Could you check a few things on this model? Use its own coordinates, in mm. Face numbers are marked on the shaded views. A direction names the side the tool comes from. Give positions to 0.01 mm unless a question says otherwise; leave off trailing zeros. Write each loop counter-clockwise with the first axis right and the second up, starting at its lowest first coordinate (ties: lowest second). Pieces come first, ordered by that corner, then holes. Notation, with made-up numbers: M -35,-34 L -5,-34 A24 ccw -5,-3 Z; hole C 68,-23 d7. An arc over 180 degrees is marked long. Write each question's results on one line, items separated by ' | '. Start each with the question number.
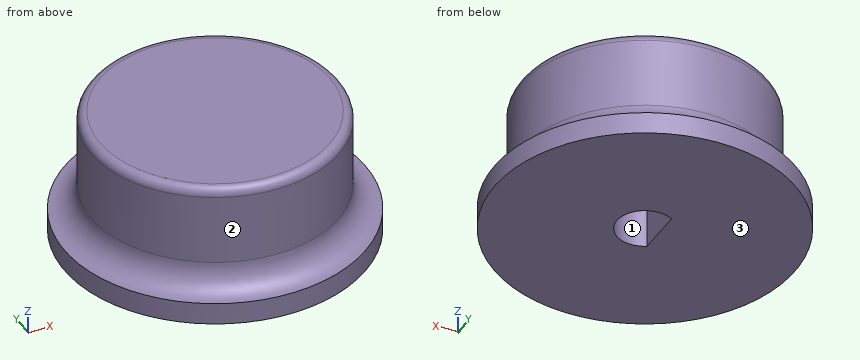
Autodesk Fusion 360 part; units mm, degrees
sketch "Sketch1" plane through (0, 0, 0) normal (0, 0, 1) x (1, 0, 0)
  line L0 (-1.45, 2.6263) -> (-1.45, -2.6263) construction
  arc A0 (-1.45, -2.6263) -> (-1.45, 2.6263) centre (0, 0) ccw construction
  arc A1 (-1.63, -2.7305) -> (-1.63, 2.7305) centre (0, 0) ccw
  line L1 (-1.63, 2.7305) -> (-1.63, -2.7305)
  circle A2 centre (0, 0) radius 17
  circle A3 centre (0, 0) radius 14
  dimension "d1" = 6
  dimension "d4" = 0.18
  dimension "d5" = 34
  dimension "d6" = 3
extrude "Extrude1" add sketch "Sketch1" along normal blind 14 contours A1 L1 | A3
extrude "Extrude2" add sketch "Sketch1" along normal blind 2 contours A2
extrude "Extrude3" cut sketch "Sketch1" along normal blind 12 contours A1 L1
fillet "Fillet1" radius 3 1 edges at (-13.0526, -5.0626, 2)
fillet "Fillet2" radius 1 1 edges at (-13.0526, -5.0626, 14)
extrude "Extrude4" add sketch "Sketch1" along normal blind 2 contours A2
extrude "Extrude5" add sketch "Sketch1" against normal blind 0.5 contours A2 | A3
equation "mountTol = 0.18 mm"
equation "d4 = mountTol"
Q1. Please list where these lines run through material, in increasing order: line 1 (Y direction, x = 0, z = 7.75); line 2 (Y direction, x = 0, z = 4); line 3 (Z direction, x = -7.5, y = -14.5). Write a range as [from, to].
Q2. For the marked faces 1, 2 and 3, which set-ups out of +Z, -Z, +X, -X, +Y, -Y let a thin tool reach every point of the face, with its end or its side?
Q3. If we section it at D-D (z = 4.25): Please give me the cut outline in (x, y).
Q4. If we section it at C-C (z = 9.5): Please give me the cut outline in (x, y).
Q5. I'm going to push flat-ended pins straight in: P1, Ø3, axis at y = -10, z = 9, coming from the +X side; P2, Ø5, axis at y = -8.5, z = 5, coming from the +X side; P3, Ø1.6, axis at y = -0.5, z = 4.5, coming from the +X side. Where does each tip first touch, or does it pass through?
Determined:
1) line 1: y = [-14, -3.18], [3.18, 14] | line 2: y = [-14.17, -3.18], [3.18, 14.17] | line 3: z = [-0.5, 2.08]
2) face 1: -Z | face 2: +Z | face 3: -Z, +X, -X, +Y, -Y
3) outline: C 0,0 d28.19; hole M -1.63,-2.73 A3.18 ccw long -1.63,2.73 Z
4) outline: C 0,0 d28; hole M -1.63,-2.73 A3.18 ccw long -1.63,2.73 Z
5) P1: stops at x = 11.12 | P2: stops at x = 13.06 | P3: stops at x = 14.29
